Source: three-view drawing plus pictorial views. Frame: mm from the lowest corner of the part. A direction names the side the tool comes from. Round coordinates to 2 decimals unless told otherwise and drop trailing zeros. Write each loop counter-clockwise with the first axis right and the second up, starting at its lowest first coordinate (ties: lowest second). Pieces come first, ordered by that corner, then holes. Notation, with made-up numbers: M 15,-5.75 L 60,-5.75 A24 ccw 60,19.25 Z; hole C 74,1.5 d7. An arc over 180 degrees is marked long. Answer as CSV lines item,"result". Start each with the question number.
Q1. Mould query, pull axis Y, two halves, no side actions, for the marked faces 1, 2 and 3. Classes: pulls with the +Y half, pulls with the -Y half, needs draft (parallel to the pull), parting line crosses it, or undercut.
Q2. Section query A-A on y = 5. Output: boundary loops of the cut face in (x, z).
Q3. Section query D-D on z = 24. Output: boundary loops of the cut face in (x, y).
Q4. Section query B-B on x = 3.5. Output: boundary loops of the cut face in (y, z).
Q5. Section query C-C on x = 20. Output: boundary loops of the cut face in (y, z), and give its area (3 significant figures).
Q6. Reachability of the marked faces 4 and 5 from +Z, -Z, +X, -X, +Y, -Y: full face, straight path, thin tool, end or side. Return the list, or none.
Q7. Ray query, probe 1 along Y at (x, z) = (20, 2.5); probe 2 along Z at (x, y) = (32.5, 29.5); probe 3 along Z at (x, y) = (14.5, 17). Return the intervals inside material, ascending.
Q8. First-contact query: pin 1 (2 mm diameter, centred on x = 32, y = 29.5, fed in from +Z); pin 2 (12 mm diameter, centred on x = 34.5, z = 23, fed in from +Y); pin 3 (3 mm diameter, centred on x = 6, z = 4.5, fed in from -Y); pin 4 (1.5 mm diameter, centred on x = 14.5, y = 18.5, fed in from +Z). Flat tips, straight axial feed; report the tip coordinate or a pass-through.
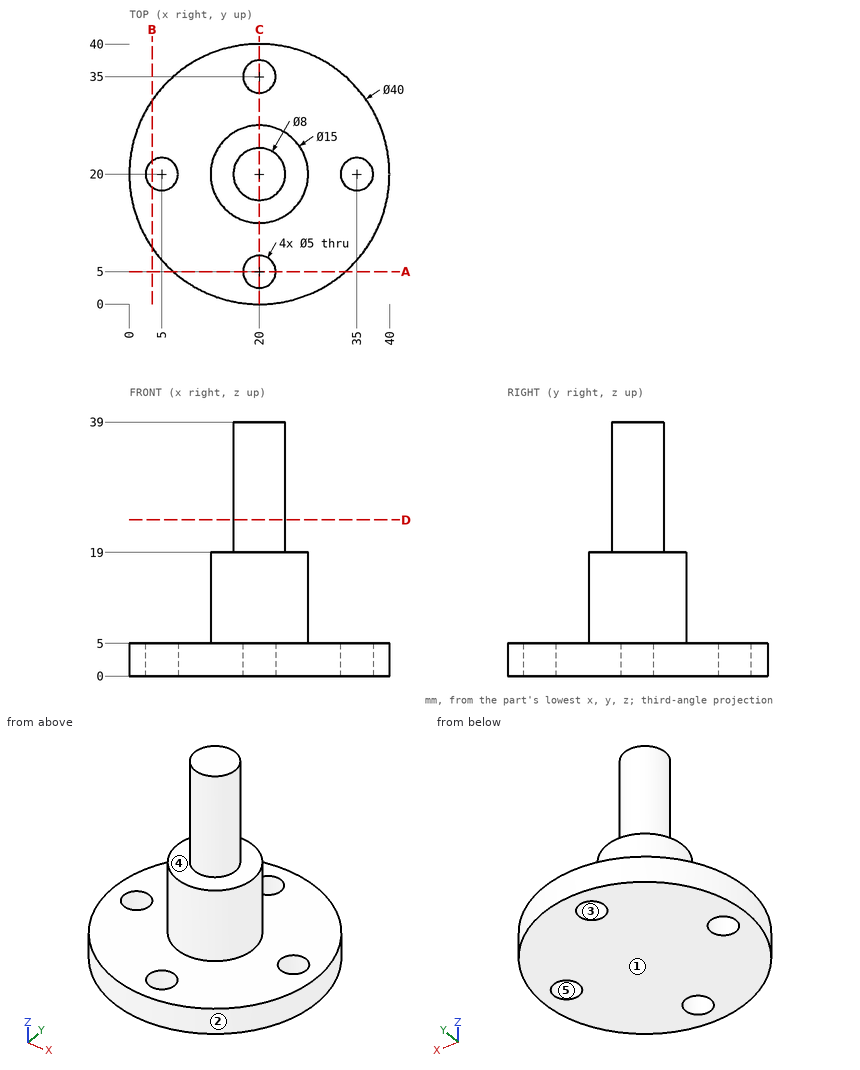
Entries:
1,face 1,"needs draft"
1,face 2,"parting line crosses it"
1,face 3,"undercut"
2,outline,"M 6.77,0 L 17.5,0 L 17.5,5 L 6.77,5 Z; M 22.5,0 L 33.23,0 L 33.23,5 L 22.5,5 Z"
3,outline,"C 20,20 d8"
4,outline,"M 8.7,0 L 18,0 L 18,5 L 8.7,5 Z; M 22,0 L 31.3,0 L 31.3,5 L 22,5 Z"
5,outline,"M 0,0 L 2.5,0 L 2.5,5 L 0,5 Z; M 7.5,0 L 32.5,0 L 32.5,5 L 27.5,5 L 27.5,19 L 24,19 L 24,39 L 16,39 L 16,19 L 12.5,19 L 12.5,5 L 7.5,5 Z; M 37.5,0 L 40,0 L 40,5 L 37.5,5 Z"
5,area,"520 mm^2"
6,face 4,"+Z"
6,face 5,"+Z, -Z"
7,probe 1,"y = 0 to 2.5, 7.5 to 32.5, 37.5 to 40"
7,probe 2,"z = 0 to 5"
7,probe 3,"z = 0 to 19"
8,pin 1,"stops at z = 5"
8,pin 2,"passes through"
8,pin 3,"stops at y = 4.39"
8,pin 4,"stops at z = 19"
